Read the model definition and answer for the solid it produces. Units are mm, in the model's axes. Face numbers are marked on the shaded views. A direction names the side the tool comes from. Give positions to 0.01 mm unless a question says otherwise; leave off trailing zeros. Order: outer loops, then holes, each group sorted by start corner. A loop starts at its lowest first (then second) coordinate and runs counter-clockwise, first axis right, second up. Notation, with made-up numbers: (9, -4) -> (40, -4) arc R24 cw to (40, 9) -> close; hole circle Ø10 at (-2, 59). An arc over 180 degrees is marked (long way). Use one line per item in the form item = value.
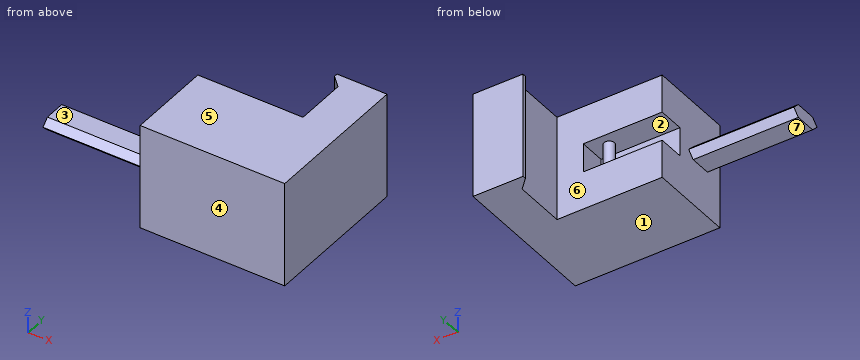
```python
from build123d import *

# Parameters (mm, degrees)
ESQUISSE1_W             = 27.5
ESQUISSE1_H             = 20
BOSS_EXTRU_1_DEPTH      = 16.19
ESQUISSE2_W             = 7.5
ESQUISSE2_H             = 20
BOSS_EXTRU_2_DEPTH      = 12.5
BOSS_EXTRU_4_DEPTH      = 20
ESQUISSE5_W             = 15
ESQUISSE5_H             = 5.5
ENL_V_MAT_EXTRU_1_DEPTH = 5
ESQUISSE11_R            = 1
BOSS_EXTRU_5_DEPTH      = 5.5
ESQUISSE12_W            = 20
ESQUISSE12_H            = 2.7
BOSS_EXTRU_6_DEPTH      = 2
CHANFREIN1_SIZE         = 2


with BuildPart() as part:
    # Esquisse1 → Boss.-Extru.1 (new body)
    with BuildSketch(Plane(origin=(0, 0, 0), x_dir=(1, 0, 0), z_dir=(0, 1, 0))):
        with Locations((13.75, 10)):
            Rectangle(ESQUISSE1_W, ESQUISSE1_H)
    extrude(amount=BOSS_EXTRU_1_DEPTH)

    # Esquisse2 → Boss.-Extru.2 (add)
    with BuildSketch(Plane(origin=(0, 16.19, 0), x_dir=(1, 0, 0), z_dir=(0, 1, 0))):
        with Locations((23.75, 10)):
            Rectangle(ESQUISSE2_W, ESQUISSE2_H)
    extrude(amount=BOSS_EXTRU_2_DEPTH)

    # Esquisse4 → Boss.-Extru.4 (add)
    with BuildSketch(Plane.ZY):
        Polygon((-8.75, 7.5), (-8.75, 3.5), (-10, 2.25), (-11.25, 3.5), (-11.25, 7.5), (-10, 8.75), align=None)
    extrude(amount=BOSS_EXTRU_4_DEPTH)

    # Esquisse5 → Enlèv. mat.-Extru.1 (cut)
    with BuildSketch(Plane(origin=(0, 16.19, 0), x_dir=(1, 0, 0), z_dir=(0, 1, 0))):
        with Locations((7.5, 10)):
            Rectangle(ESQUISSE5_W, ESQUISSE5_H)
    extrude(amount=-ENL_V_MAT_EXTRU_1_DEPTH, mode=Mode.SUBTRACT)

    # Esquisse11 → Boss.-Extru.5 (add)
    with BuildSketch(Plane.XY.offset(-12.75)):
        with Locations(Location((11.77506405, 13.69, 0), (0, 0, 180))):
            Circle(ESQUISSE11_R)
    extrude(amount=BOSS_EXTRU_5_DEPTH)

    # Esquisse12 → Boss.-Extru.6 (add)
    with BuildSketch(Plane.ZY.offset(-20)):
        with Locations((-10, 27.34)):
            Rectangle(ESQUISSE12_W, ESQUISSE12_H)
    extrude(amount=BOSS_EXTRU_6_DEPTH)

    # Chanfrein1
    chanfrein1_edges = [part.edges().sort_by_distance(p)[0] for p in [
        (18, 25.99, -10),
    ]]
    chamfer(chanfrein1_edges, length=CHANFREIN1_SIZE - 0.0001)  # a hair under: the kernel refuses the full size


solid = part.part
```
Item 1: Straight lines are drawn through the part: L1, parallel to X at y = 17.75, z = -6.75; L2, parallel to Z at x = 4, y = 13; L3, parallel to Y at x = 13, z = -2.5. For each, find the intervals that lie inside material, in ascending order. Write a range as from..to.
Checks:
L1 = 20..27.5
L2 = -20..-12.75, -7.25..0
L3 = 0..16.19
Item 2: Given pin 1 Ø4 at (x, y) = (10, 14) entering from +Z; pin 2 Ø10 at (x, y) = (-7, 21.5) entering from +Z; pin 3 Ø10 at (x, y) = (-15, 8.5) entering from +Z; pin 4 Ø3 at (x, y) = (-15, 5.5) entering from -Z, each flat-ended and moving along its own axis, determine where each tip first touches the part or whether it passes through.
Checks:
pin_1 = 0
pin_2 = through
pin_3 = -8.75
pin_4 = -11.25
Item 3: The part is cut by section C-C on y = 13.69. Give the vertices of the cut face in (x, z).
Checks:
outline = (0, -20) -> (27.5, -20) -> (27.5, 0) -> (0, 0) -> (0, -7.25) -> (10.78, -7.25) -> (10.78, -12.75) -> (0, -12.75) -> close; hole (12.78, -12.75) -> (15, -12.75) -> (15, -7.25) -> (12.78, -7.25) -> close
Item 4: Which of the six approach directions +Z, -Z, +X, -X, +Y, -Y give full straight-line access (tool end or side, diameter ignored) to the marked faces 5, 6 and 7?
Checks:
face_5 = +Z, +X, -X, +Y, -Y
face_6 = +Z, -Z, -X
face_7 = -Z, -X, +Y, -Y
Item 5: Determine the mould class of the marked faces 1, 2, 3 and 4 for opening direction Z: +Z half, -Z half, draft (parallel to the pull), parting line (faces both ways), or undercut.
Checks:
face_1 = -Z half
face_2 = undercut
face_3 = +Z half
face_4 = draft
Item 6: The part is cut by section B-B on x = 4.5. Give the vertices of the cut face in (y, z).
Checks:
outline = (0, -20) -> (16.19, -20) -> (16.19, -12.75) -> (11.19, -12.75) -> (11.19, -7.25) -> (16.19, -7.25) -> (16.19, 0) -> (0, 0) -> close
